```python
from build123d import *

# Parameters (mm, degrees)
SKETCH_1_W          = 106.4
SKETCH_1_H          = 108.6
EXTRUDE_1_DEPTH     = 1
SKETCH_2_W          = 103.5
SKETCH_2_H          = 105.7
SKETCH_2_W_2        = 102.1
SKETCH_2_H_2        = 104.3
EXTRUDE_2_DEPTH     = 2.5
SKETCH_4_R          = 1.8
CUT_EXTRUDE_1_DEPTH = 77.098488815
SKETCH_13_R         = 4.2
SKETCH_13_R_2       = 1.8
EXTRUDE_8_DEPTH     = 15.89
SKETCH_14_W         = 89
SKETCH_14_H         = 101.449206074
CUT_EXTRUDE_6_DEPTH = 15.89


with BuildPart() as part:
    # 草图1 → 凸台-拉伸1 (new body)
    with BuildSketch(Plane(origin=(0, 0, 0), x_dir=(1, 0, 0), z_dir=(0, 1, 0))):
        Rectangle(SKETCH_1_W, SKETCH_1_H)
    extrude(amount=EXTRUDE_1_DEPTH)

    # 草图2 → 凸台-拉伸2 (add)
    with BuildSketch(Plane.XZ):
        Rectangle(SKETCH_2_W, SKETCH_2_H)
        Rectangle(SKETCH_2_W_2, SKETCH_2_H_2, mode=Mode.SUBTRACT)
    extrude(amount=EXTRUDE_2_DEPTH)

    # 草图4 → 切除-拉伸1 (cut, through all)
    with BuildSketch(Plane(origin=(0, 1, 0), x_dir=(1, 0, 0), z_dir=(0, 1, 0))):
        with Locations(Location((47.5, 44.5, 0), (0, 0, 270))):
            Circle(SKETCH_4_R)
        with Locations(Location((-47.5, 44.5, 0), (0, 0, 270))):
            Circle(SKETCH_4_R)
        with Locations(Location((-47.5, -45.5, 0), (0, 0, 270))):
            Circle(SKETCH_4_R)
        with Locations(Location((47.5, -45.5, 0), (0, 0, 270))):
            Circle(SKETCH_4_R)
    extrude(amount=-CUT_EXTRUDE_1_DEPTH, mode=Mode.SUBTRACT)

    # 草图13 → 凸台-拉伸8 (add)
    # profile 1 of 4: a face of its own
    with BuildSketch(Plane.XZ):
        with Locations(Location((-47.5, 45.5, 0), (0, 0, 147.697454791))):
            Circle(SKETCH_13_R)
        with Locations(Location((-47.5, 45.5, 0), (0, 0, 90))):
            Circle(SKETCH_13_R_2, mode=Mode.SUBTRACT)
    # profile 2 of 4: a face of its own
    with BuildSketch(Plane.XZ):
        with Locations(Location((47.5, 45.5, 0), (0, 0, 32.302545209))):
            Circle(SKETCH_13_R)
        with Locations(Location((47.5, 45.5, 0), (0, 0, 90))):
            Circle(SKETCH_13_R_2, mode=Mode.SUBTRACT)
    # profile 3 of 4: a face of its own
    with BuildSketch(Plane.XZ):
        with Locations(Location((-47.5, -44.5, 0), (0, 0, 147.697454791))):
            Circle(SKETCH_13_R)
        with Locations(Location((-47.5, -44.5, 0), (0, 0, 90))):
            Circle(SKETCH_13_R_2, mode=Mode.SUBTRACT)
    # profile 4 of 4: a face of its own
    with BuildSketch(Plane.XZ):
        with Locations(Location((47.5, -44.5, 0), (0, 0, 32.302545209))):
            Circle(SKETCH_13_R)
        with Locations(Location((47.5, -44.5, 0), (0, 0, 90))):
            Circle(SKETCH_13_R_2, mode=Mode.SUBTRACT)
    extrude(amount=EXTRUDE_8_DEPTH)

    # 草图14 → 切除-拉伸6 (cut)
    with BuildSketch(Plane.XZ.offset(15.89)):
        Rectangle(SKETCH_14_W, SKETCH_14_H)
    extrude(amount=-CUT_EXTRUDE_6_DEPTH, mode=Mode.SUBTRACT)


solid = part.part
```
Read the model definition and answer for the solid it produces. Units are mm, in the model's axes. A direction names the side the tool comes from. Round coordinates to 2 decimals unless told otherwise and drop trailing zeros. Loops run counter-clockwise (first coordinate to the right, second up) from the corner with the lowest first, then second, coordinate; pieces in that order, holes last. Notation, with made-up numbers: (-32, 58.5) -> (13, 58.5) arc R22 ccw to (13, 74.5) -> close; hole circle Ø7 at (39.5, 21.5). An arc over 180 degrees is marked (long way). One line per item, written item: value.
1) A cutting plane is placed at A-A (y = -5). Determine the outline of the cut face in (x, z), and give its area (3 significant figures).
Answer list:
outline: (-44.5, -47.44) -> (-44.5, -41.56) arc R4.2 ccw (long way) to start; (-44.5, 42.56) -> (-44.5, 48.44) arc R4.2 ccw (long way) to start; (44.5, -47.44) arc R4.2 ccw (long way) to (44.5, -41.56) -> close; (44.5, 42.56) arc R4.2 ccw (long way) to (44.5, 48.44) -> close; hole circle Ø3.6 at (-47.5, -44.5); hole circle Ø3.6 at (-47.5, 45.5); hole circle Ø3.6 at (47.5, -44.5); hole circle Ø3.6 at (47.5, 45.5)
area: 162 mm²
2) The mould has two halves that part along Z. Classify faces 1 (the face through (49, -15.89, -43)), 2 (the face through (-1, -1, -52.85)), 3 (the face through (51.05, -1, 0)): pulls with the +Z half, pulls with the -Z half, needs draft (parallel to the pull), parting line crosses it, or undercut.
Answer list:
face 1: needs draft
face 2: pulls with the -Z half
face 3: undercut
3) A cutting plane is placed at D-D (x = -33). Determine the outline of the cut face in (y, z).
Answer list:
outline: (-2.5, -52.85) -> (0, -52.85) -> (0, -54.3) -> (1, -54.3) -> (1, 54.3) -> (0, 54.3) -> (0, 52.85) -> (-2.5, 52.85) -> (-2.5, 52.15) -> (0, 52.15) -> (0, -52.15) -> (-2.5, -52.15) -> close
4) Consider L1, parallel to Z at x = 47.5, y = -4; L2, parallel to X at y = -4.5, z = 45.5; L3, parallel to X at y = -2.25, z = 29. Determine where each line is inside the solid, lowest interval first. Write a range as [from, to].
Answer list:
L1: z = [-48.7, -46.3], [-42.7, -40.3], [41.3, 43.7], [47.3, 49.7]
L2: x = [-51.7, -49.3], [-45.7, -44.5], [44.5, 45.7], [49.3, 51.7]
L3: x = [-51.75, -51.05], [51.05, 51.75]
5) Flat-ended cylindrical pins translate along their axes: P1, Ø0.8, axis at y = -1.5, z = -10, coming from the -X side; P2, Ø4.5, axis at x = -47.5, z = 45.5, coming from the -Y side; P3, Ø8, axis at x = 15, z = -25, coming from the -Y side; P4, Ø6.5, axis at y = -4.5, z = -45, coming from the +X side. Find the tip coordinate at first contact, or state that the pin passes through.
Answer list:
P1: stops at x = -51.75
P2: stops at y = -15.89
P3: stops at y = 0
P4: stops at x = 51.75
6) For faces 4 (the face through (-1, 1, -1)), 5 (the face through (-1, 0, -1)), 6 (the face through (51.75, -1, -1)), 7 (the face through (-51.75, -1, -1)), determine the directions among +Z, -Z, +X, -X, +Y, -Y from which every point of the face is accessible in a straight line to the end or side of a thin tool.
Answer list:
face 4: +Z, -Z, +X, -X, +Y
face 5: -Y
face 6: +Z, -Z, +X, -Y
face 7: +Z, -Z, -X, -Y
7) A cutting plane is placed at C-C (z = -44.5). Determine the outline of the cut face in (x, y).
Answer list:
outline: (-53.2, 0) -> (-51.75, 0) -> (-51.75, -2.5) -> (-51.7, -2.5) -> (-51.7, -15.89) -> (-49.3, -15.89) -> (-49.3, 1) -> (-53.2, 1) -> close; (-45.7, -15.89) -> (-44.5, -15.89) -> (-44.5, 0) -> (44.5, 0) -> (44.5, -15.89) -> (45.7, -15.89) -> (45.7, 1) -> (-45.7, 1) -> close; (49.3, -15.89) -> (51.7, -15.89) -> (51.7, -2.5) -> (51.75, -2.5) -> (51.75, 0) -> (53.2, 0) -> (53.2, 1) -> (49.3, 1) -> close
8) A cutting plane is placed at B-B (x = -47.5). Determine the outline of the cut face in (y, z).
Answer list:
outline: (-15.89, -48.7) -> (0, -48.7) -> (0, -52.15) -> (-2.5, -52.15) -> (-2.5, -52.85) -> (0, -52.85) -> (0, -54.3) -> (1, -54.3) -> (1, -46.3) -> (-15.89, -46.3) -> close; (-15.89, -42.7) -> (1, -42.7) -> (1, 43.7) -> (-15.89, 43.7) -> (-15.89, 41.3) -> (0, 41.3) -> (0, -40.3) -> (-15.89, -40.3) -> close; (-15.89, 47.3) -> (1, 47.3) -> (1, 54.3) -> (0, 54.3) -> (0, 52.85) -> (-2.5, 52.85) -> (-2.5, 52.15) -> (0, 52.15) -> (0, 49.7) -> (-15.89, 49.7) -> close
